Read the model definition and answer for the solid it produces. Units are mm, in the model's axes. A direction names the side the tool comes from. Give positions to 0.01 mm unless a question says otherwise; leave off trailing zeros. Order: outer loops, then holes, each group sorted by start corner. A loop starts at its lowest first (then second) coordinate and runs counter-clockwise, first axis right, second up.
Item 1: Which of the six approach directions +Z, -Z, +X, -X, +Y, -Y give full straight-line access (tool end or side, diameter ignored) to faces 1 (the face through (-12, -13, 1)), 2 (the face through (-3, 16, 1)), 3 (the face through (-12, 13, 1)), 4 (the face through (5.967, -8.715, 1.521))?
Item 2: Find the intervals of material crossed by line 1 along X through (y, z) = (6, 1.5); line 2 along Y through (x, z) = (1.5, 0.9); line 3 along Y through (x, z) = (-9.5, 2.4), in increasing order.
Item 3: Given pin 1 Ø1.5 at (y, z) = (16, 1) entering from -X; pin 2 Ø1 at (x, z) = (-1, 0.5) entering from +Y; pin 3 Ø1 at (x, y) = (8, 3) entering from +Z; pin 4 Ø4 at (x, y) = (-6, -4.5) entering from +Z, each flat-ended and moving along its own axis, determine where each tip first touches the part or whether it passes through.
Item 4: A cutting plane is placed at C-C (x = -10.5). Write down the section's boundary in (y, z).
Item 5: A cutting plane is placed at D-D (z = 1.5). State how many separate pieces and enclosed holes the cut face has, plus the area to 3 significant figures.
Item 6: A cutting plane is placed at B-B (y = 0). Write down the section's boundary in (x, z), plus the area to 3 significant figures.
Item 7: A cutting plane is placed at A-A (y = -14.5). Write down the section's boundary in (x, z).
Item 8: The mould has two halves that part along Y. Classify faces 5 (the face through (8, -9, 1)), 6 (the face through (0, -13, 1)), 7 (the face through (3, 0, 0)): +Y half, -Y half, draft (parallel to the pull), parting line (faces both ways), or undercut.
from build123d import *

# Parameters (mm, degrees)
SKETCH_1_W      = 5.333333333
SKETCH_1_H      = 18
SKETCH_1_W_2    = 5.333333334
EXTRUDE_1_DEPTH = 3
FILLET_2_R      = 1


with BuildPart() as part:
    # 草图1 → 凸台-拉伸1 (new body)
    with BuildSketch(Plane.XY):
        Polygon((-11, 19.5), (-11, 13), (-13, 13), (-13, -13), (-11, -13), (-11, -19.5), (-3, -19.5), (-3, -13), (3, -13), (3, -19.5), (11, -19.5), (11, -13), (13, -13), (13, 13), (11, 13), (11, 19.5), (3, 19.5), (3, 13), (-3, 13), (-3, 19.5), align=None)
        with Locations((8.333333334, 0)):
            Rectangle(SKETCH_1_W, SKETCH_1_H, mode=Mode.SUBTRACT)
        with Locations((-8.333333334, 0)):
            Rectangle(SKETCH_1_W, SKETCH_1_H, mode=Mode.SUBTRACT)
        Rectangle(SKETCH_1_W_2, SKETCH_1_H, mode=Mode.SUBTRACT)
    extrude(amount=EXTRUDE_1_DEPTH)

    # 圆角2
    fillet_2_edges = [part.edges().sort_by_distance(p)[0] for p in [
        (5.666666667, 9, 1.5),
        (5.666666667, -9, 1.5),
        (11, -9, 1.5),
        (11, 9, 1.5),
        (-11, 9, 1.5),
        (-11, -9, 1.5),
        (-5.666666667, -9, 1.5),
        (-5.666666667, 9, 1.5),
        (-2.666666667, 9, 1.5),
        (-2.666666667, -9, 1.5),
        (2.666666667, -9, 1.5),
        (2.666666667, 9, 1.5),
    ]]
    fillet(fillet_2_edges, radius=FILLET_2_R)


solid = part.part
Response values:
1. face 1: +Z, -Z, -X, -Y
1. face 2: +Z, -Z, +Y
1. face 3: +Z, -Z, -X, +Y
1. face 4: +Z, -Z
2. line 1: x = -13 to -11, -5.67 to -2.67, 2.67 to 5.67, 11 to 13
2. line 2: y = -13 to -9, 9 to 13
2. line 3: y = -19.5 to -9, 9 to 19.5
3. pin 1: stops at x = -11
3. pin 2: stops at y = 13
3. pin 3: passes through
3. pin 4: stops at z = 3
4. outline: (-19.5, 0) - (-8.87, 0) - (-8.87, 3) - (-19.5, 3) - close; (8.87, 0) - (19.5, 0) - (19.5, 3) - (8.87, 3) - close
5. separate pieces: 1
5. enclosed holes: 3
5. area: 599 mm2
6. outline: (-13, 0) - (-11, 0) - (-11, 3) - (-13, 3) - close; (-5.67, 0) - (-2.67, 0) - (-2.67, 3) - (-5.67, 3) - close; (2.67, 0) - (5.67, 0) - (5.67, 3) - (2.67, 3) - close; (11, 0) - (13, 0) - (13, 3) - (11, 3) - close
6. area: 30.0 mm2
7. outline: (-11, 0) - (-3, 0) - (-3, 3) - (-11, 3) - close; (3, 0) - (11, 0) - (11, 3) - (3, 3) - close
8. face 5: undercut
8. face 6: -Y half
8. face 7: draft
